from build123d import *

# Parameters (mm, degrees)
SKETCH033_R     = 5
PAD018_DEPTH    = 20
SKETCH034_R     = 3.5
POCKET016_DEPTH = 0.5
SKETCH037_R     = 4.5
POCKET018_DEPTH = 1
FILLET003_R     = 0.5


with BuildPart() as part:
    # Sketch033 → Pad018 (new body)
    with BuildSketch(Plane.XY):
        Circle(SKETCH033_R)
    extrude(amount=PAD018_DEPTH)

    # Sketch034 (on Face3 of Pad018) → Pocket016 (cut)
    with BuildSketch(Plane.XY.offset(20)):
        Circle(SKETCH034_R)
    extrude(amount=-POCKET016_DEPTH, mode=Mode.SUBTRACT)

    # Sketch037 (on Face5 of Pocket016) → Pocket018 (cut)
    with BuildSketch(Plane.XY.offset(19.5)):
        Circle(SKETCH037_R)
    extrude(amount=-POCKET018_DEPTH, mode=Mode.SUBTRACT)

    # Fillet003
    fillet003_edges = [part.edges().sort_by_distance(p)[0] for p in [
        (-5, 0, 20),
    ]]
    fillet(fillet003_edges, radius=FILLET003_R)


solid = part.part
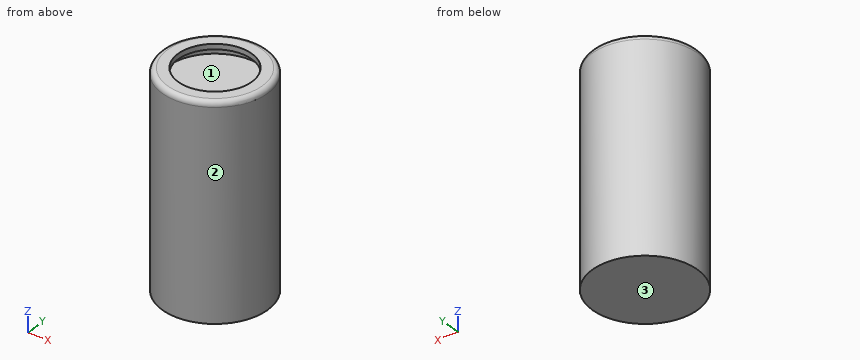
The listing builds one solid part. Answer for the finished solid, in the listing's coordinates (mm). Face numbers are marked on the shaded views. Coordinates: 2 decimals unless noted, no trailing zeros. Order: outer loops, then holes, each group sorted by start corner. A loop starts at its lowest first (then second) coordinate and runs counter-clockwise, first axis right, second up. Notation, with made-up numbers: M 60,86.25 L 111,86.25 A33 cw 111,117.25 Z; hole C -12,-35.5 d10. An arc over 180 degrees is marked long. Use CSV: the item, a comma, the result in double quotes.
Q1. Straight lines are drawn through the part: L1, parallel to Z at x = -1.5, y = 3.5; L2, parallel to Y at x = 0, z = 18.9; L3, parallel to Z at x = -2, y = 0. For each, find the intervals that lie inside material, in ascending order.
Here are the results:
L1,"0 to 18.5, 19.5 to 20"
L2,"-5 to -4.5, 4.5 to 5"
L3,"0 to 18.5"
Q2. Determine the mould class of the marked faces 1, 2 and 3 for opening direction Y: pulls with the +Y half, pulls with the -Y half, needs draft (parallel to the pull), parting line crosses it, or undercut.
Here are the results:
face 1,"undercut"
face 2,"parting line crosses it"
face 3,"needs draft"
Q3. Section A-A (x = 0) is taken. Determine the outline of the cut face in (y, z), then the cut area to 3 significant figures.
Here are the results:
outline,"M -5,0 L 5,0 L 5,19.5 A0.5 ccw 4.5,20 L 3.5,20 L 3.5,19.5 L 4.5,19.5 L 4.5,18.5 L -4.5,18.5 L -4.5,19.5 L -3.5,19.5 L -3.5,20 L -4.5,20 A0.5 ccw -5,19.5 Z"
area,"187 mm2"
Q4. Given pin 1 Ø4.5 at (x, y) = (0, 0.5) entering from +Z; pin 2 Ø1.5 at (y, z) = (-1.5, 11) entering from -X; pin 3 Ø4 at (y, z) = (2.5, 7.5) entering from +X, each flat-ended and moving along its own axis, determine where each tip first touches the part or whether it passes through.
Here are the results:
pin 1,"z = 18.5"
pin 2,"x = -4.94"
pin 3,"x = 4.97"
